Autodesk Inventor part; units mm, degrees
ref_plane "YZ Plane" through (0, 0, 0) normal (1, 0, 0) x (0, 1, 0)
ref_plane "XZ Plane" through (0, 0, 0) normal (0, 1, 0) x (-1, 0, 0)
ref_plane "XY Plane" through (0, 0, 0) normal (0, 0, 1) x (1, 0, 0)
sketch "Sketch1" plane through (0, 0, 0) normal (0, 1, 0) x (-1, 0, 0)
  line L0 (0, 2.4651) -> (7.9791, 2.4651)
  line L1 (7.9791, 2.4651) -> (7.9791, 0)
  line L2 (0, 0) -> (-2.7044, 0)
  line L3 (-2.7044, 0) -> (-5.1567, 1.3844)
  line L4 (-5.1567, 1.3844) -> (0, 2.4651)
  line L5 (7.9791, 0) -> (-2.7044, 0)
extrude "Extrusion1" add sketch "Sketch1" along normal blind 2.54
extrude "Extrusion2" [suppressed]
sketch "Sketch2" plane through (0, 2.54, 0) normal (0, 1, 0) x (1, 0, 0)
  line L0 (0, -2.4651) -> (2.2705, -0.7352)
  line L1 (0.3368, -2.2085) -> (0.3368, -0.1091)
  line L2 (2.2705, -0.7352) -> (0, 0)
  line L3 (1.4116, -0.4571) -> (1.4116, -1.3896)
  line L4 (0.3368, -2.2085) -> (1.4116, -1.3896)
  line L5 (0.3368, -0.1091) -> (1.4116, -0.4571)
  line L6 (0.3368, -2.2085) -> (1.4116, -1.3896)
extrude "Extrusion3" cut sketch "Sketch2" against normal blind 1.27 contours L1 L2 L3 L0
sketch "Sketch3" plane through (-7.9791, 0, 2.4651) normal (0, 0, 1) x (1, 0, 0)
  circle A0 centre (1.4488, 1.319) radius 0.9757
  point P0 (7.9791, 0)
extrude "Extrusion4" cut sketch "Sketch3" against normal blind 5.08
properties part number "hook" material "Nylon 6/6"
Read the model definition and answer for the solid it produces. Units are mm, in the model's axes. A direction names the side the tool comes from. Give positions to 0.01 mm unless a question says otherwise; leave off trailing zeros. Loops run counter-clockwise (first coordinate to the right, second up) from the corner with the lowest first, then second, coordinate; pieces in that order, holes last.
Item 1: The part is cut by section A-A (y = 0.55). Write down the section's boundary in (x, z), and give its area (3 significant figures).
Item 2: For faces 1 (the flat face through (-7.979, 1, 1)), 2 (the flat face through (0.882, 1.914, 0.286)), determine the directions among +Z, -Z, +X, -X, +Y, -Y from which every point of the face is accessible in a straight line to the end or side of a thin tool.
Item 3: The part is cut by section C-C (x = -7). Write down the section's boundary in (y, z).
Item 4: The part is cut by section D-D (y = 1.15). Write down the section's boundary in (x, z), and give its area (3 significant figures).
Item 5: The part is cut by section B-B (z = 1.25). Write down the section's boundary in (x, y).
Item 6: Find the intervals of material crossed by line 1 along X through (y, z) = (1.45, 0.9); line 2 along X through (y, z) = (2.15, 0.55); line 3 along Y through (x, z) = (0.5, 0.3), in increasing order.
Item 7: This flat-tipped pin is pushed along its axis until it touches: pin 1 Ø1 at (y, z) = (1.5, 1.5) entering from +X. Where does it stop, or does it pass through?
Item 8: The mould has two halves that part along Z. Classify faces 3 (the flat face through (1, 1.27, 1)), 4 (the cylindrical face through (-6.08, 0.453, 1.25)), 5 (the flat face through (-3, 1, 0)): released by +Z, released by -Z, zero draft, split by the parting line, or undercut.
Taken from the geometry:
1. outline: (-7.98, 0) - (-7.13, 0) - (-7.13, 2.47) - (-7.98, 2.47) - close; (-5.93, 0) - (2.7, 0) - (5.16, 1.38) - (0, 2.47) - (-5.93, 2.47) - close
1. area: 24.9 mm2
2. face 1: +Z, -Z, -X, +Y, -Y
2. face 2: +Y
3. outline: (0, 0) - (0.46, 0) - (0.46, 2.47) - (0, 2.47) - close; (2.17, 0) - (2.54, 0) - (2.54, 2.47) - (2.17, 2.47) - close
4. outline: (-7.98, 0) - (-7.49, 0) - (-7.49, 2.47) - (-7.98, 2.47) - close; (-5.57, 0) - (2.7, 0) - (5.16, 1.38) - (0, 2.47) - (-5.57, 2.47) - close
4. area: 23.2 mm2
5. outline: (-7.98, 0) - (4.92, 0) - (4.92, 2.54) - (1.41, 2.54) - (1.41, 1.27) - (0.34, 1.27) - (0.34, 2.54) - (-7.98, 2.54) - close; hole circle Ø1.95 at (-6.53, 1.32)
6. line 1: x = -7.98 to -7.5, -5.56 to 0.34, 1.41 to 4.3
6. line 2: x = -7.98 to -7.04, -6.02 to 0.34, 1.41 to 3.68
6. line 3: y = 0 to 1.27
7. pin 1: stops at x = 5.16
8. face 3: undercut
8. face 4: zero draft
8. face 5: released by -Z
